Here's how the part is built. I have some questions about the finished solid (model axes, mm). A direction names the side the tool comes from. Round coordinates to 2 decimals unless told otherwise and drop trailing zeros. Order: outer loops, then holes, each group sorted by start corner. A loop starts at its lowest first (then second) coordinate and runs counter-clockwise, first axis right, second up.
```python
from build123d import *

# Parameters (mm, degrees)
F0_W     = 27
F0_H     = 27
F0_R     = 2
F0_R_2   = 4
F5_DEPTH = 2
F3_R     = 2
F3_R_2   = 4
F6_DEPTH = 2
F4_R     = 2
F7_DEPTH = 2
F8_R     = 2
F9_R     = 2


with BuildPart() as f5:
    # F0 (on Top) → F5 (new body)
    with BuildSketch(Plane.XY):
        Rectangle(F0_W, F0_H)
        with Locations((-5.656854, -5.656854)):
            Circle(F0_R, mode=Mode.SUBTRACT)
        with Locations((0, -8)):
            Circle(F0_R, mode=Mode.SUBTRACT)
        with Locations((5.656854, -5.656854)):
            Circle(F0_R, mode=Mode.SUBTRACT)
        with Locations((-8, 0)):
            Circle(F0_R, mode=Mode.SUBTRACT)
        with Locations((-5.656854, 5.656854)):
            Circle(F0_R, mode=Mode.SUBTRACT)
        Circle(F0_R_2, mode=Mode.SUBTRACT)
        with Locations((5.656854, 5.656854)):
            Circle(F0_R, mode=Mode.SUBTRACT)
        with Locations((8, 0)):
            Circle(F0_R, mode=Mode.SUBTRACT)
        with Locations((0, 8)):
            Circle(F0_R, mode=Mode.SUBTRACT)
    extrude(amount=F5_DEPTH)

    # F3 (on face) → F6 (join)
    with BuildSketch(Plane(origin=(-13.5, 0, 0), x_dir=(0, -1, 0), z_dir=(-1, 0, 0))):
        with BuildLine():
            Line((-13.5, 17), (-13.5, 0))
            Line((-13.5, 0), (13.5, 0))
            Line((13.5, 0), (13.5, 17))
            ThreePointArc((13.5, 17), (0, 29), (-13.5, 17))
        make_face()
        with Locations((-5.656854, 9.343146)):
            Circle(F3_R, mode=Mode.SUBTRACT)
        with Locations((0, 7)):
            Circle(F3_R, mode=Mode.SUBTRACT)
        with Locations((5.656854, 9.343146)):
            Circle(F3_R, mode=Mode.SUBTRACT)
        with Locations((-8, 15)):
            Circle(F3_R, mode=Mode.SUBTRACT)
        with Locations((-5.656854, 20.656854)):
            Circle(F3_R, mode=Mode.SUBTRACT)
        with Locations((0, 15)):
            Circle(F3_R_2, mode=Mode.SUBTRACT)
        with Locations((5.656854, 20.656854)):
            Circle(F3_R, mode=Mode.SUBTRACT)
        with Locations((8, 15)):
            Circle(F3_R, mode=Mode.SUBTRACT)
        with Locations((0, 23)):
            Circle(F3_R, mode=Mode.SUBTRACT)
    extrude(amount=-F6_DEPTH)

    # F4 (on face) → F7 (join)
    with BuildSketch(Plane(origin=(13.5, 0, 0), x_dir=(0, -1, 0), z_dir=(-1, 0, 0))):
        with BuildLine():
            Line((-13.5, 0), (13.5, 0))
            Line((13.5, 0), (13.5, 17))
            ThreePointArc((13.5, 17), (0, 29), (-13.5, 17))
            Line((-13.5, 17), (-13.5, 0))
        make_face()
        with Locations((-5.656854, 9.343146)):
            Circle(F4_R, mode=Mode.SUBTRACT)
        with BuildLine():
            ThreePointArc((2, 7), (-1.414214, 5.585786), (0, 9))
            ThreePointArc((0, 9), (1.414214, 8.414214), (2, 7))
        make_face(mode=Mode.SUBTRACT)
        with Locations((5.656854, 9.343146)):
            Circle(F4_R, mode=Mode.SUBTRACT)
        with Locations((-8, 15)):
            Circle(F4_R, mode=Mode.SUBTRACT)
        with Locations((-5.656854, 20.656854)):
            Circle(F4_R, mode=Mode.SUBTRACT)
        with BuildLine():
            ThreePointArc((4, 15), (2.828427, 12.171573), (0, 11))
            ThreePointArc((0, 11), (-2.828427, 17.828427), (4, 15))
        make_face(mode=Mode.SUBTRACT)
        with Locations((5.656854, 20.656854)):
            Circle(F4_R, mode=Mode.SUBTRACT)
        with Locations((8, 15)):
            Circle(F4_R, mode=Mode.SUBTRACT)
        with Locations((0, 23)):
            Circle(F4_R, mode=Mode.SUBTRACT)
    extrude(amount=F7_DEPTH)

    # F8
    f8_edges = [f5.edges().sort_by_distance(p)[0] for p in [
        (-13.5, 0, 0),
    ]]
    fillet(f8_edges, radius=F8_R)

    # F9
    f9_edges = [f5.edges().sort_by_distance(p)[0] for p in [
        (13.5, 0, 0),
    ]]
    fillet(f9_edges, radius=F9_R)


solid = f5.part
```
1. On a 3-axis mill with a long thin cutter (end or side, diameter ignored), from which of +Z, -Z, +X, -X, +Y, -Y can I reach the whole of each face in a straight line? I mean faces 4 (the flat face through (-13.5, 0, 10)), 5 (the flat face through (-3, 3, 2)). Say none if no direction works.
Evaluation:
face 4: +Z, -Z, -X, +Y, -Y
face 5: +Z, +Y, -Y
2. If we section it at C-C, the plane x = 3.25: Write out the boundary of the cut face in (y, z), and give its area (3 significant figures).
Evaluation:
outline: (-13.5, 0) - (-2.33, 0) - (-2.33, 2) - (-13.5, 2) - close; (2.33, 0) - (13.5, 0) - (13.5, 2) - (2.33, 2) - close
area: 44.7 mm2
3. If we section it at B-B, the plane z = 3.75: Write out the boundary of the cut face in (x, y).
Evaluation:
outline: (-13.5, -13.5) - (-11.5, -13.5) - (-11.5, 13.5) - (-13.5, 13.5) - close; (11.5, -13.5) - (13.5, -13.5) - (13.5, 13.5) - (11.5, 13.5) - close
4. I need wall thicknesses on probe 1 along Y at (x, z) = (0, 1.1); probe 2 along X at (y, z) = (-6, 11.5); probe 3 along Z at (x, y) = (-12.2, 0). Which ranges of each line are inside material? Lowest first, please.
Evaluation:
probe 1: y = -13.5 to -10, -6 to -4, 4 to 6, 10 to 13.5
probe 2: x = -13.5 to -11.5, 11.5 to 13.5
probe 3: z = 0.13 to 5, 9 to 11, 19 to 21, 25 to 29
5. If we section it at A-A, the plane x = 0: Write out the boundary of the cut face in (y, z), and give its area (3 significant figures).
Evaluation:
outline: (-13.5, 0) - (-10, 0) - (-10, 2) - (-13.5, 2) - close; (-6, 0) - (-4, 0) - (-4, 2) - (-6, 2) - close; (4, 0) - (6, 0) - (6, 2) - (4, 2) - close; (10, 0) - (13.5, 0) - (13.5, 2) - (10, 2) - close
area: 22.0 mm2
6. I'm going to push flat-ended pins straight in: P1, Ø2.5, axis at x = -5.66, y = -5.66, coming from the +Z side; P2, Ø1, axis at x = -3.5, y = -4, coming from the +Z side. Where does each tip first touch, or does it pass through?
Evaluation:
P1: passes through
P2: stops at z = 2
7. If we mould it in two halves opening along X, with no side actions, what happens to faces 1 (the cylindrical face through (-12.514, 0.521, 18.966)), 2 (the cylindrical face through (-12.93, 0.19, 0.6)), 3 (the cylindrical face through (-4.7, 3.9, 1))? For each: released by +X, released by -X, zero draft, split by the parting line, or undercut.
Evaluation:
face 1: zero draft
face 2: released by -X
face 3: undercut
8. If we section it at D-D, the plane y = 8.75: Write out the boundary of the cut face in (x, z), and give its area (3 significant figures).
Evaluation:
outline: (-13.5, 2) arc R2 ccw to (-11.5, 0) - (-1.85, 0) - (-1.85, 2) - (-11.5, 2) - (-11.5, 13.15) - (-13.5, 13.15) - close; (-13.5, 16.85) - (-11.5, 16.85) - (-11.5, 25.81) - (-13.5, 25.81) - close; (1.85, 0) - (11.5, 0) arc R2 ccw to (13.5, 2) - (13.5, 13.15) - (11.5, 13.15) - (11.5, 2) - (1.85, 2) - close; (11.5, 16.85) - (13.5, 16.85) - (13.5, 25.81) - (11.5, 25.81) - close
area: 125 mm2
